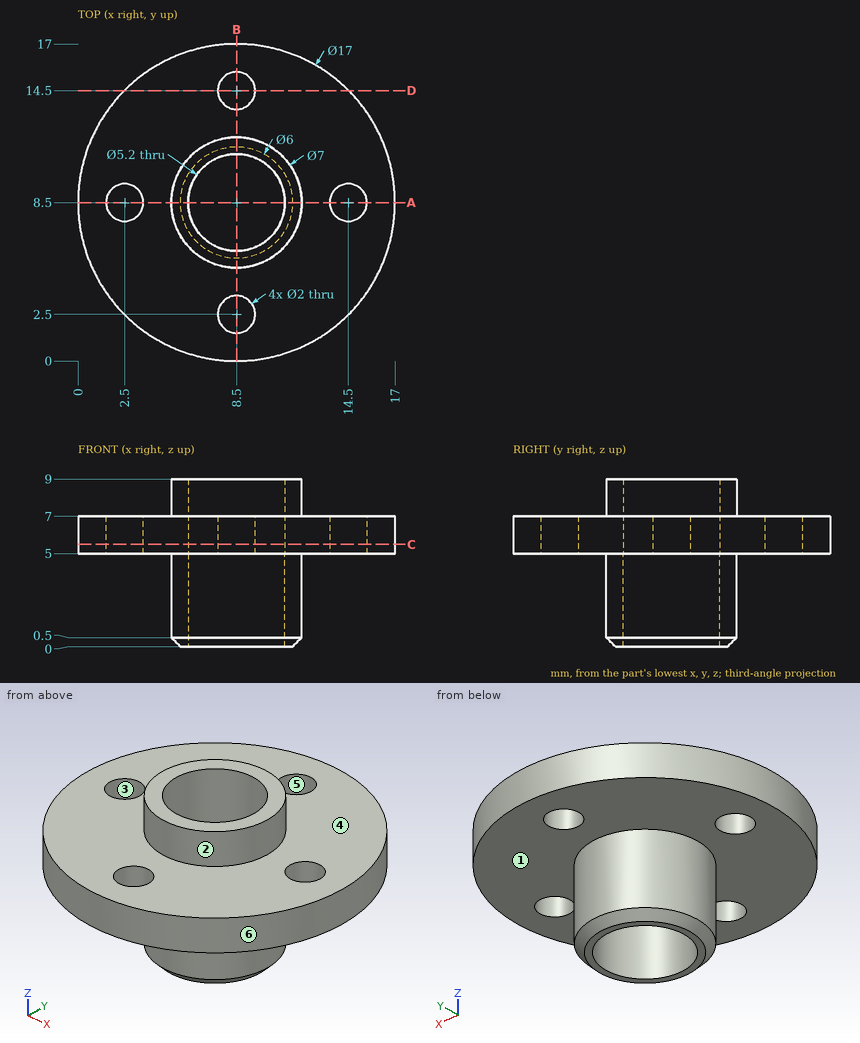
Design review of the part shown in the three views and the two pictorial views. Dimensions are in mm from the part's minimum x, y and z. A direction names the side the tool comes from. Give positions to 0.01 mm unless a question says otherwise; leave off trailing zeros. Write each loop counter-clockwise with the first axis right and the second up, starting at its lowest first coordinate (ties: lowest second). Pieces come first, ordered by that corner, then holes.
Item 1: Take a section at A-A (y = 8.5). Give the boundary of the cut face in (x, z).
Item 2: Insertion check: P1, Ø4.5, axis at x = 8.5, y = 8.5, coming from the +Z side; P2, Ø1, axis at x = 4, y = 14.5, coming from the +Z side; P3, Ø6, axis at x = 4.5, y = 13.5, coming from the -Z side; P4, Ø2, axis at y = 9, z = 6, coming from the -X side. Each pin has a flat end and moves straight along its axis. Give the tip position at first contact, or say it passes through.
Item 3: Take a section at C-C (z = 5.5). Give the boundary of the cut face in (x, y), and give its area (3 significant figures).
Item 4: The part is to be moulded in two halves that separate along X. For the marked faces 4, 5 and 6, say which applies: +X half, -X half, draft (parallel to the pull), parting line (faces both ways), or undercut.
Item 5: Machinability: for the marked faces 1, 2 and 3, which of the approach directions +Z, -Z, +X, -X, +Y, -Y give a long, thin tool a straight path to every point of the face, cutting with its end or side? Answer none if there is none.
Item 6: Take a section at D-D (y = 14.5). Give the boundary of the cut face in (x, z).
Item 7: Wall thickness on probe 1 along Y at (x, z) = (8.5, 5.9); probe 2 along Y at (x, z) = (8, 6); probe 3 along Y at (x, z) = (8.5, 7.55): over which ranges is each line inside the solid? List them lowest first.
Established:
1. outline: (0, 5) - (1.5, 5) - (1.5, 7) - (0, 7) - close; (3.5, 5) - (5, 5) - (5, 0.5) - (5.5, 0) - (5.9, 0) - (5.9, 9) - (5, 9) - (5, 7) - (3.5, 7) - close; (11.1, 0) - (11.5, 0) - (12, 0.5) - (12, 5) - (13.5, 5) - (13.5, 7) - (12, 7) - (12, 9) - (11.1, 9) - close; (15.5, 5) - (17, 5) - (17, 7) - (15.5, 7) - close
2. P1: passes through
2. P2: stops at z = 7
2. P3: stops at z = 0.4
2. P4: stops at x = 0
3. outline: circle Ø17 at (8.5, 8.5); hole circle Ø2 at (2.5, 8.5); hole circle Ø5.2 at (8.5, 8.5); hole circle Ø2 at (8.5, 2.5); hole circle Ø2 at (8.5, 14.5); hole circle Ø2 at (14.5, 8.5)
3. area: 193 mm2
4. face 4: draft
4. face 5: undercut
4. face 6: parting line
5. face 1: -Z
5. face 2: +Z
5. face 3: +Z, -Z
6. outline: (2.48, 5) - (7.5, 5) - (7.5, 7) - (2.48, 7) - close; (9.5, 5) - (14.52, 5) - (14.52, 7) - (9.5, 7) - close
7. probe 1: y = 0 to 1.5, 3.5 to 5.9, 11.1 to 13.5, 15.5 to 17
7. probe 2: y = 0.01 to 1.63, 3.37 to 5.95, 11.05 to 13.63, 15.37 to 16.99
7. probe 3: y = 5 to 5.9, 11.1 to 12
